Work out the finished part from the listing and answer in its coordinate system (mm). Round coordinates to 2 decimals unless told otherwise and drop trailing zeros. Loops run counter-clockwise (first coordinate to the right, second up) from the corner with the lowest first, then second, coordinate; pieces in that order, holes last. Notation, with made-up numbers: M 12,37 L 22,37 A12 cw 22,44 Z; hole C 13,29.5 d6. An arc over 180 degrees is marked long. One line per item, written item: value.
```python
from build123d import *

# Parameters (mm, degrees)
AUFSATZ_LINEAR_AUSTRAGEN1_DEPTH      = 15
AUFSATZ_LINEAR_AUSTRAGEN1_DEPTH_BACK = 15
SKIZZE1_R                            = 2.55


with BuildPart() as part:
    # Skizze1 → Aufsatz-Linear austragen1 (new, two sides: drawn at the far end of the back side and taken through both)
    with BuildSketch(Plane(origin=(0, 0, 0), x_dir=(1, 0, 0), z_dir=(0, 1, 0)).offset(-AUFSATZ_LINEAR_AUSTRAGEN1_DEPTH_BACK)):
        with BuildLine():
            Line((0, 7), (35, 7))
            ThreePointArc((35, 7), (42, 0), (35, -7))
            Line((35, -7), (0, -7))
            ThreePointArc((0, -7), (-7, 0), (0, 7))
        make_face()
        with Locations(Location((0, 0, 0), (0, 0, 270))):
            Circle(SKIZZE1_R, mode=Mode.SUBTRACT)
    extrude(amount=AUFSATZ_LINEAR_AUSTRAGEN1_DEPTH + AUFSATZ_LINEAR_AUSTRAGEN1_DEPTH_BACK)


solid = part.part
```
1) Find section A-A (z = 0). Give the vertices of the cut face in (x, y), then the cut area to 3 significant figures.
Check values:
outline: M -7,-15 L -2.55,-15 L -2.55,15 L -7,15 Z; M 2.55,-15 L 42,-15 L 42,15 L 2.55,15 Z
area: 1,320 mm2
2) Find the intervals of material crossed by probe 1 along X at (y, z) = (-8.25, 0); probe 2 along X at (y, z) = (7.75, -1); probe 3 along Z at (x, y) = (-4, -2.5), in increasing order. Write a range as from..to.
Check values:
probe 1: -7..-2.55, 2.55..42
probe 2: -6.93..-2.35, 2.35..41.93
probe 3: -5.74..5.74
3) Find section C-C (z = -4.5). Give the vertices of the cut face in (x, y).
Check values:
outline: M -5.36,-15 L 40.36,-15 L 40.36,15 L -5.36,15 Z
4) Find section B-B (y = -5.75). Give the vertices of the cut face in (x, z).
Check values:
outline: M 0,-7 L 35,-7 A7 ccw 35,7 L 0,7 A7 ccw Z; hole C 0,0 d5.1
5) The mould has two halves that part along X. Classify faces 1 (the face through (17, 0, -7)), 2 (the face through (42, 0, 0)), 3 (the face through (0.77, -0.21, 2.43)): +X half, -X half, draft (parallel to the pull), parting line (faces both ways), or undercut.
Check values:
face 1: draft
face 2: +X half
face 3: undercut
6) This flat-tipped pin is pushed along its axis until it touches: pin 1 (6 mm diameter, centred on y = -6.5, z = -5, fed in from +X). Where does it stop, or does it pass through?
Check values:
pin 1: x = 41.71
